Answer from the drawing. Dimensions are ordinates in mm from the lowest x, y and z of the part. A direction names the side the tool comes from. Coordinates: 2 decimals unless noted, no trailing zeros. Order: outer loops, then holes, each group sorted by start corner. A loop starts at its lowest first (then second) coordinate and runs counter-clockwise, first axis right, second up. Notation, with made-up numbers: (83, -25) - (137, -25) arc R14 ccw to (137, -20) - close; hole circle Ø4 at (72, 46). An arc over 180 degrees is marked (long way). One line per item, written item: value. Start each with the question number.
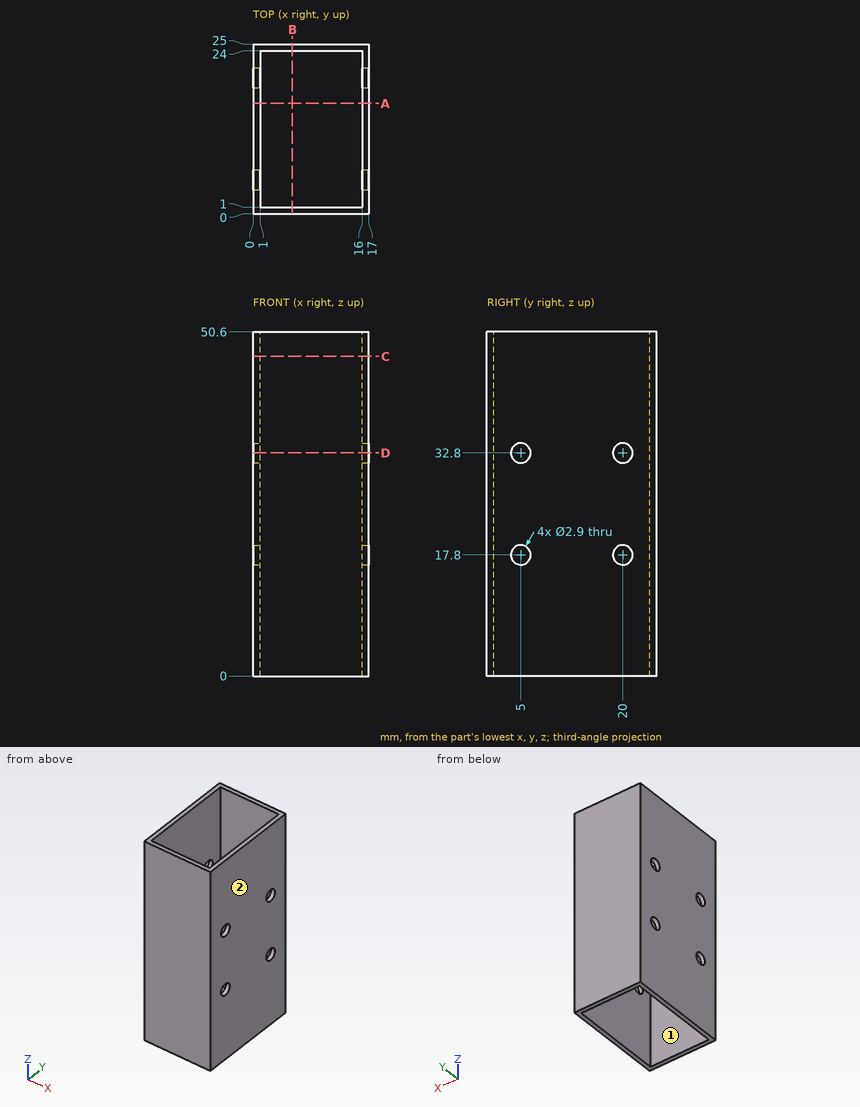
(1) For the marked faces 1 and 2, determine the directions among +Z, -Z, +X, -X, +Y, -Y from which every point of the face is accessible in a straight line to the end or side of a thin tool.
(2) The part is cut by section B-B on x = 5.75. Determine the outline of the cut face in (y, z), plus the area to 3 significant figures.
(3) The part is cut by section D-D on z = 32.8. Determine the outline of the cut face in (x, y), plus the area to 3 significant figures.
(4) The part is cut by section C-C on z = 47. Determine the outline of the cut face in (x, y), plus the area to 3 significant figures.
(5) Consider probe 1 along Z at (x, y) = (16.65, 5); probe 2 along Y at (x, z) = (16.75, 17.8); probe 3 along Y at (x, z) = (4, 21). Determine where each line is inside the solid, lowest interval first.
(6) The part is cut by section A-A on y = 16.25. Determine the outline of the cut face in (x, z).
Completed:
1. face 1: +Z, -Z
1. face 2: +Z, -Z, +X, +Y, -Y
2. outline: (0, 0) - (1, 0) - (1, 50.6) - (0, 50.6) - close; (24, 0) - (25, 0) - (25, 50.6) - (24, 50.6) - close
2. area: 101 mm2
3. outline: (0, 0) - (17, 0) - (17, 3.55) - (16, 3.55) - (16, 1) - (1, 1) - (1, 3.55) - (0, 3.55) - close; (0, 6.45) - (1, 6.45) - (1, 18.55) - (0, 18.55) - close; (0, 21.45) - (1, 21.45) - (1, 24) - (16, 24) - (16, 21.45) - (17, 21.45) - (17, 25) - (0, 25) - close; (16, 6.45) - (17, 6.45) - (17, 18.55) - (16, 18.55) - close
3. area: 68.4 mm2
4. outline: (0, 0) - (17, 0) - (17, 25) - (0, 25) - close; hole (1, 1) - (16, 1) - (16, 24) - (1, 24) - close
4. area: 80.0 mm2
5. probe 1: z = 0 to 16.35, 19.25 to 31.35, 34.25 to 50.6
5. probe 2: y = 0 to 3.55, 6.45 to 18.55, 21.45 to 25
5. probe 3: y = 0 to 1, 24 to 25
6. outline: (0, 0) - (1, 0) - (1, 50.6) - (0, 50.6) - close; (16, 0) - (17, 0) - (17, 50.6) - (16, 50.6) - close
